CAD build for the part. Positions are in the model's coordinates, mm. Face numbers are marked on the shaded views. A direction names the side the tool comes from. Round coordinates to 2 decimals unless told otherwise and drop trailing zeros. Order: outer loops, then holes, each group sorted by start corner. A loop starts at its lowest first (then second) coordinate and runs counter-clockwise, first axis right, second up.
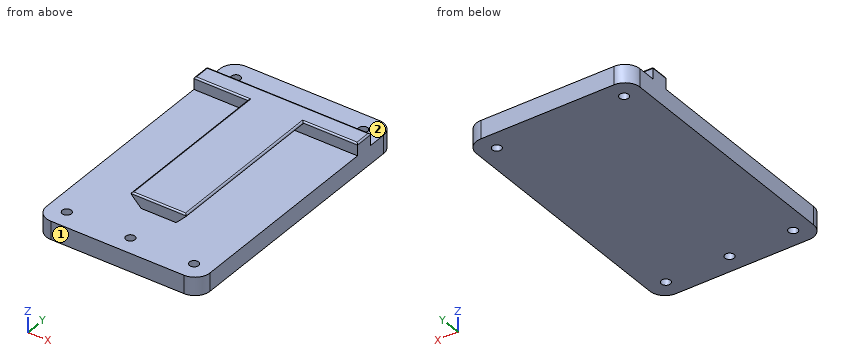
```python
from build123d import *

# Parameters (mm, degrees)
F0_W      = 54
F0_H      = 90
F1_DEPTH  = 10
F3_DEPTH  = 73
F5_D      = 3
F6_W      = 11
F6_H      = 4
F7_DEPTH  = 54.001
F8_R      = 5
F9_W      = 19.5
F9_H      = 19
F9_R      = 1.5
F10_DEPTH = 4
F11_R     = 0.5


with BuildPart() as f1:
    # F0 (on Top) → F1 (new body)
    with BuildSketch(Plane.XY):
        Rectangle(F0_W, F0_H)
    extrude(amount=F1_DEPTH)

    # F2 (on face) → F3 (cut)
    with BuildSketch(Plane.XZ.offset(45)):
        Polygon((-27, 10), (-27, 6), (-5.75, 6), (-9.75, 10), align=None)
        Polygon((5.75, 6), (27, 6), (27, 10), (9.75, 10), align=None)
    extrude(amount=-F3_DEPTH, mode=Mode.SUBTRACT)

    # F5 (through all)
    with Locations(Plane(origin=(0, 0, 0), x_dir=(1, 0, 0), z_dir=(0, 0, -1))):
        with Locations((-21, 39), (21, 39), (21, -39), (-21, -39), (0, 39)):
            Hole(F5_D / 2)

    # F6 (on face) → F7 (cut, through all)
    with BuildSketch(Plane.YZ.offset(27)):
        with Locations((39.5, 8)):
            Rectangle(F6_W, F6_H)
    extrude(amount=-F7_DEPTH, mode=Mode.SUBTRACT)

    # F8
    f8_edges = [f1.edges().sort_by_distance(p)[0] for p in [
        (27, -45, 3),
        (27, 45, 3),
        (-27, 45, 3),
        (-27, -45, 3),
    ]]
    fillet(f8_edges, radius=F8_R)

    # F9 (on face) → F10 (cut)
    with BuildSketch(Plane.XY.offset(10)):
        with Locations((0, -35.5)):
            Rectangle(F9_W, F9_H)
        with Locations((0, -39)):
            Circle(F9_R, mode=Mode.SUBTRACT)
    extrude(amount=-F10_DEPTH, mode=Mode.SUBTRACT)

    # F11
    f11_edges = [f1.edges().sort_by_distance(p)[0] for p in [
        (-9.75, 1, 10),
        (9.75, 1, 10),
        (-18.375, 28, 10),
        (18.375, 28, 10),
        (0, -26, 10),
        (-27, 31, 10),
        (0, 34, 10),
        (27, 31, 10),
    ]]
    fillet(f11_edges, radius=F11_R)


solid = f1.part
```
1. Tool access for the marked faces 1 and 2: list every direction of +Z, -Z, +X, -X, +Y, -Y with a clear straight run to the whole face (end or side of a thin tool).
2. Drill centre lines: line 1 (Y direction, x = -21, z = 1.95); line 2 (X direction, y = 39, z = 4.4); line 3 (X direction, y = -39, z = 2.85). Where is each one in solid material? Low to high.
3. Cut at C-C, the plane y = -1.5. Write the cut outline in (x, z).
4. Cut at D-D, the plane z = 7. Write the cut outline in (x, y).
5. Cut at B-B, the plane x = 21. Write the cut outline in (y, z).
6. Pin check, flat tips, straight feed: P1, Ø5.5, axis at x = 2, y = 37, coming from the +Z side; P2, Ø1.8, axis at x = -2, z = 8, coming from the -Y side; P3, Ø1.8, axis at x = -5, z = 7.5, coming from the +Y side; P4, Ø2.5, axis at x = 0, y = -39, coming from the -Z side. Stop position of each tip, or through.
7. Cut at A-A, the plane y = -39. Write the cut outline in (x, z), and give its area (3 significant figures).
Outcome:
1. face 1: +Z, -Z, +X, -X, -Y
1. face 2: +Z, +X, -X, +Y
2. line 1: y = -45 to -40.5, -37.5 to 37.5, 40.5 to 45
2. line 2: x = -27 to -22.5, -19.5 to 19.5, 22.5 to 27
2. line 3: x = -27 to -22.5, -19.5 to -1.5, 1.5 to 19.5, 22.5 to 27
3. outline: (-27, 0) - (27, 0) - (27, 6) - (5.75, 6) - (8.9, 9.15) arc R0.5 ccw to (8.54, 10) - (-8.54, 10) arc R0.5 ccw to (-8.9, 9.15) - (-5.75, 6) - (-27, 6) - close
4. outline: (-27, 28) - (-6.75, 28) - (-6.75, -26) - (6.75, -26) - (6.75, 28) - (27, 28) - (27, 34) - (-27, 34) - close
5. outline: (-45, 0) - (-40.5, 0) - (-40.5, 6) - (-45, 6) - close; (-37.5, 0) - (37.5, 0) - (37.5, 6) - (34, 6) - (34, 9.5) arc R0.5 ccw to (33.5, 10) - (28.5, 10) arc R0.5 ccw to (28, 9.5) - (28, 6) - (-37.5, 6) - close; (40.5, 0) - (45, 0) - (45, 6) - (40.5, 6) - close
6. P1: stops at z = 6
6. P2: stops at y = -26
6. P3: stops at y = 34
6. P4: passes through
7. outline: (-27, 0) - (-22.5, 0) - (-22.5, 6) - (-27, 6) - close; (-19.5, 0) - (-1.5, 0) - (-1.5, 6) - (-19.5, 6) - close; (1.5, 0) - (19.5, 0) - (19.5, 6) - (1.5, 6) - close; (22.5, 0) - (27, 0) - (27, 6) - (22.5, 6) - close
7. area: 270 mm2
